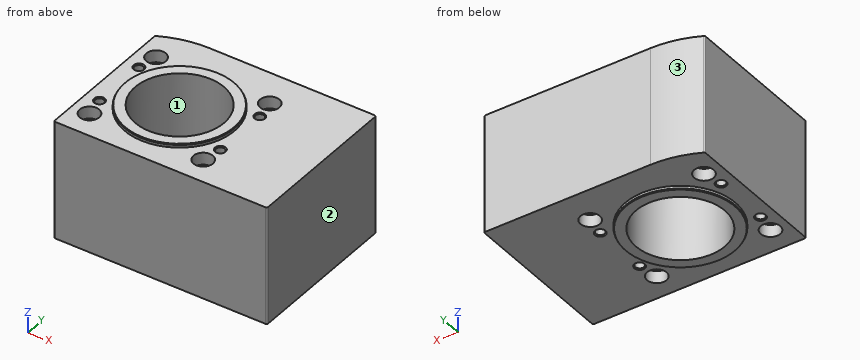
from build123d import *

# Parameters (mm, degrees)
LINEAR_AUSTRAGEN1_DEPTH = 66.5
SKIZZE3_R               = 25
LINEAR_AUSTRAGEN2_DEPTH = 70.5


with BuildPart() as part:
    # Skizze1 → Linear austragen1 (new body)
    with BuildSketch(Plane.XY):
        with BuildLine():
            Line((-42, 39.959083258), (-42, -40.5))
            ThreePointArc((-42, -40.5), (-41.707106781, -41.207106781), (-41, -41.5))
            Line((-41, -41.5), (77, -41.5))
            ThreePointArc((77, -41.5), (77.707106781, -41.207106781), (78, -40.5))
            Line((78, -40.5), (78, 46))
            ThreePointArc((78, 46), (77.707106781, 46.707106781), (77, 47))
            Line((77, 47), (-15.7, 47))
            ThreePointArc((-15.7, 47), (-28.937844321, 45.441495991), (-41.451785714, 40.851209745))
            ThreePointArc((-41.451785714, 40.851209745), (-41.851993461, 40.482635684), (-42, 39.959083258))
        make_face()
    extrude(amount=LINEAR_AUSTRAGEN1_DEPTH)

    # Skizze2 → Rotation1 (revolve)
    with BuildSketch(Plane(origin=(0, 0, 0), x_dir=(0, 0, -1), z_dir=(1, 0, 0))):
        Polygon((-68.5, 0), (-68.5, 30.711324865), (-68, 31), (1.5, 31), (2, 30.711324865), (2, 0), align=None)
    revolve(axis=Axis((0, 0, -2), (0, 0, 1)))

    # Skizze3 → Linear austragen2 (cut)
    with BuildSketch(Plane.XY.offset(-2)):
        Circle(SKIZZE3_R)
    extrude(amount=LINEAR_AUSTRAGEN2_DEPTH, mode=Mode.SUBTRACT)

    # Skizze4 → Schnitt-Rotation1 (revolve, cut)
    with BuildSketch(Plane(origin=(-32, 0, 0), x_dir=(0, 0, -1), z_dir=(1, 0, 0))):
        Polygon((-68.5, 27), (-68.5, 32.5), (-59.7, 32.5), (-59.7, 30.3), (-6.8, 30.3), (-6.8, 32.5), (2, 32.5), (2, 27), align=None)
    revolve(axis=Axis((-32, 27, -2), (0, 0, 1)), mode=Mode.SUBTRACT)

    # Skizze5 → Schnitt-Rotation2 (revolve, cut)
    with BuildSketch(Plane(origin=(-32, 0, 0), x_dir=(0, 0, -1), z_dir=(1, 0, 0))):
        Polygon((-68.5, -27), (-68.5, -21.5), (-59.7, -21.5), (-59.7, -23.7), (-6.8, -23.7), (-6.8, -21.5), (2, -21.5), (2, -27), align=None)
    revolve(axis=Axis((-32, -27, -2), (0, 0, 1)), mode=Mode.SUBTRACT)

    # Skizze6 → Schnitt-Rotation3 (revolve, cut)
    with BuildSketch(Plane(origin=(32, 0, 0), x_dir=(0, 0, -1), z_dir=(1, 0, 0))):
        Polygon((-68.5, -27), (-68.5, -21.5), (-59.7, -21.5), (-59.7, -23.7), (-6.8, -23.7), (-6.8, -21.5), (2, -21.5), (2, -27), align=None)
    revolve(axis=Axis((32, -27, -2), (0, 0, 1)), mode=Mode.SUBTRACT)

    # Skizze7 → Schnitt-Rotation4 (revolve, cut)
    with BuildSketch(Plane(origin=(32, 0, 0), x_dir=(0, 0, -1), z_dir=(1, 0, 0))):
        Polygon((-68.5, 27), (-68.5, 32.5), (-59.7, 32.5), (-59.7, 30.3), (-6.8, 30.3), (-6.8, 32.5), (2, 32.5), (2, 27), align=None)
    revolve(axis=Axis((32, 27, -2), (0, 0, 1)), mode=Mode.SUBTRACT)

    # Skizze8 → Schnitt-Rotation5 (revolve, cut)
    with BuildSketch(Plane(origin=(34, 0, 0), x_dir=(0, 0, -1), z_dir=(1, 0, 0))):
        Polygon((-18.519415637, 16), (-17.1, 18.4585), (-0.5415, 18.4585), (0, 19), (0, 16), align=None)
    revolve(axis=Axis((34, 16, 0), (0, 0, 1)), mode=Mode.SUBTRACT)

    # Skizze9 → Schnitt-Rotation6 (revolve, cut)
    with BuildSketch(Plane(origin=(34, 0, 0), x_dir=(0, 0, -1), z_dir=(1, 0, 0))):
        Polygon((-18.519415637, -16), (-17.1, -13.5415), (-0.5415, -13.5415), (0, -13), (0, -16), align=None)
    revolve(axis=Axis((34, -16, 0), (0, 0, 1)), mode=Mode.SUBTRACT)

    # Skizze10 → Schnitt-Rotation7 (revolve, cut)
    with BuildSketch(Plane(origin=(-34, 0, 0), x_dir=(0, 0, -1), z_dir=(1, 0, 0))):
        Polygon((-18.519415637, 16), (-17.1, 18.4585), (-0.5415, 18.4585), (0, 19), (0, 16), align=None)
    revolve(axis=Axis((-34, 16, 0), (0, 0, 1)), mode=Mode.SUBTRACT)

    # Skizze11 → Schnitt-Rotation8 (revolve, cut)
    with BuildSketch(Plane(origin=(-34, 0, 0), x_dir=(0, 0, -1), z_dir=(1, 0, 0))):
        Polygon((-18.519415637, -16), (-17.1, -13.5415), (-0.5415, -13.5415), (0, -13), (0, -16), align=None)
    revolve(axis=Axis((-34, -16, 0), (0, 0, 1)), mode=Mode.SUBTRACT)

    # Skizze12 → Schnitt-Rotation9 (revolve, cut)
    with BuildSketch(Plane(origin=(-34, 0, 0), x_dir=(0, 0, -1), z_dir=(1, 0, 0))):
        Polygon((-66.5, 16), (-66.5, 19), (-65.9585, 18.4585), (-49.4, 18.4585), (-47.980584363, 16), align=None)
    revolve(axis=Axis((-34, 16, 47.980584363), (0, 0, 1)), mode=Mode.SUBTRACT)

    # Skizze13 → Schnitt-Rotation10 (revolve, cut)
    with BuildSketch(Plane(origin=(-34, 0, 0), x_dir=(0, 0, -1), z_dir=(1, 0, 0))):
        Polygon((-66.5, -16), (-66.5, -13), (-65.9585, -13.5415), (-49.4, -13.5415), (-47.980584363, -16), align=None)
    revolve(axis=Axis((-34, -16, 47.980584363), (0, 0, 1)), mode=Mode.SUBTRACT)

    # Skizze14 → Schnitt-Rotation11 (revolve, cut)
    with BuildSketch(Plane(origin=(34, 0, 0), x_dir=(0, 0, -1), z_dir=(1, 0, 0))):
        Polygon((-66.5, 16), (-66.5, 19), (-65.9585, 18.4585), (-49.4, 18.4585), (-47.980584363, 16), align=None)
    revolve(axis=Axis((34, 16, 47.980584363), (0, 0, 1)), mode=Mode.SUBTRACT)

    # Skizze15 → Schnitt-Rotation12 (revolve, cut)
    with BuildSketch(Plane(origin=(34, 0, 0), x_dir=(0, 0, -1), z_dir=(1, 0, 0))):
        Polygon((-66.5, -16), (-66.5, -13), (-65.9585, -13.5415), (-49.4, -13.5415), (-47.980584363, -16), align=None)
    revolve(axis=Axis((34, -16, 47.980584363), (0, 0, 1)), mode=Mode.SUBTRACT)


solid = part.part
Input: part model. Units: mm. Frame: model coordinates. Face numbers are marked on the shaded views. Give positions to 0.01 mm unless a question says otherwise; leave off trailing zeros. Write each loop counter-clockwise with the first axis right and the second up, starting at its lowest first coordinate (ties: lowest second). Pieces come first, ordered by that corner, then holes. Notation, with made-up numbers: M 12.25,-40 L 36.25,-40 A19 ccw 36.25,-34 Z; hole C -1,83 d5. An arc over 180 degrees is marked long. Use one line per item in the form item = value.
1. Mould query, pull axis Y, two halves, no side actions, for the marked faces 1, 2 and 3. Classes: released by +Y, released by -Y, zero draft, split by the parting line, or undercut.
Outcome:
face_1 = undercut
face_2 = zero draft
face_3 = released by +Y
2. Ray query, L1, parallel to X at y = -27, z = 65; L2, parallel to Y at x = 32, z = 34; L3, parallel to X at y = 27, z = 33. Return the intervals inside material, ascending.
Outcome:
L1 = -42 to -37.5, -26.5 to 26.5, 37.5 to 78
L2 = -41.5 to -30.3, -23.7 to 23.7, 30.3 to 47
L3 = -42 to -35.3, -28.7 to 28.7, 35.3 to 78
3. Cut plane C-C on y = -28.5. State how many separate pieces and enclosed holes the cut face has, and give its area (3 significant figures).
Outcome:
separate_pieces = 3
enclosed_holes = 0
area = 7,170 mm²
4. Cut plane B-B on x = 51.5. Return loops of the section in (y, z), and give its area (3 significant figures).
Outcome:
outline = M -41.5,0 L 47,0 L 47,66.5 L -41.5,66.5 Z
area = 5,890 mm²
5. Cut plane A-A on y = 0. Return loops of the section in (x, z), and give its area (3 significant figures).
Outcome:
outline = M -42,0 L -31,0 L -31,-1.5 L -30.71,-2 L -25,-2 L -25,68.5 L -30.71,68.5 L -31,68 L -31,66.5 L -42,66.5 Z; M 25,-2 L 30.71,-2 L 31,-1.5 L 31,0 L 78,0 L 78,66.5 L 31,66.5 L 31,68 L 30.71,68.5 L 25,68.5 Z
area = 4,700 mm²
6. First-contact query: P1, Ø4, axis at x = 65, y = 2, coming from the -Z side; P2, Ø8, axis at x = 34, y = -16, coming from the +Z side; P3, Ø4.5, axis at x = 34, y = -16, coming from the +Z side. Flat tips, straight axial feed; report the tip coordinate or a pass-through.
Outcome:
P1 = 0
P2 = 66.5
P3 = 49.28
